from build123d import *

# Parameters (mm, degrees)
F1_DEPTH = 88.9
F2_DEPTH = 6.35
F3_DEPTH = 12.7
F0_W     = 25.2763175084
F0_H     = 38.1


with BuildPart() as f1:
    # F0 (on Front) → F1 (new body, symmetric)
    with BuildSketch(Plane.XZ):
        Polygon((31.75, 22.225), (-50.8, 22.225), (-50.8, -22.225), (50.8, -22.225), (50.8, 22.225), align=None)
    extrude(amount=F1_DEPTH, both=True)

    # F0 (on Front) → F2 (join, symmetric)
    with BuildSketch(Plane.XZ):
        with BuildLine():
            add(Edge.make_bspline(
                [(-50.8, 22.225), (-50.420176295, 53.6387471007), (-0.3042402085, 78.7179242207), (69.217346781, 79.3697470119)],
                knots=[0, 0, 0, 0, 133.0977115432, 133.0977115432, 133.0977115432, 133.0977115432], degree=3))
            Line((-50.8, 22.225), (31.75, 22.225))
            Line((31.75, 22.225), (31.75, 41.275))
            ThreePointArc((31.75, 41.275), (42.6864758578, 67.9911553405), (69.217346781, 79.3697470119))
        make_face()
    extrude(amount=F2_DEPTH, both=True)

    # F0 (on Front) → F3 (join, symmetric)
    with BuildSketch(Plane.XZ):
        with BuildLine():
            Line((31.75, 41.275), (31.75, 22.225))
            Line((31.75, 22.225), (50.8, 22.225))
            Line((50.8, 22.225), (50.8, 41.275))
            ThreePointArc((50.8, 41.275), (56.3796158184, 54.7453841816), (69.85, 60.325))
            Line((69.85, 60.325), (93.4907073213, 60.325))
            Line((93.4907073213, 60.325), (93.4907073213, 79.375))
            Line((93.4907073213, 79.375), (69.85, 79.375))
            add(Edge.make_bspline(
                [(69.217346781, 79.3697470119), (69.4280532127, 79.3717225603), (69.6389379005, 79.3734737242), (69.85, 79.375)],
                knots=[133.0977115432, 133.0977115432, 133.0977115432, 133.0977115432, 133.5011048643, 133.5011048643, 133.5011048643, 133.5011048643], degree=3))
            ThreePointArc((69.217346781, 79.3697470119), (42.6864758578, 67.9911553405), (31.75, 41.275))
        make_face()
        Polygon((118.732270607, 79.375), (93.4907073213, 79.375), (93.4907073213, 60.325), (119.0067035424, 60.325), align=None)
    extrude(amount=F3_DEPTH, both=True)

    # F0 (on Front) → F4 (revolve)
    with BuildSketch(Plane.XZ):
        with Locations((131.6525485671, 70.3345479765)):
            Rectangle(F0_W, F0_H)
    revolve(axis=Axis((119.0143898129, 0, 70.3345479765), (0, 0, 1)))


solid = f1.part
Work out the finished part from the listing and answer in its coordinate system (mm). A direction names the side the tool comes from. Round coordinates to 2 decimals unless told otherwise and drop trailing zeros. Order: outer loops, then holes, each group sorted by start corner. A loop starts at its lowest first (then second) coordinate and runs counter-clockwise, first axis right, second up. Notation, with made-up numbers: M -26.75,3.5 L 4.25,3.5 A33 ccw 4.25,39.5 Z; hole C 51.5,50.5 d10. An arc over 180 degrees is marked long. Put each result on its own line as item: value. Start each with the question number.
Q1. Section A-A, the plane x = 78 is taken. Write down the section's boundary in (y, z) (3 decimals).
Q2. Flat-ended cylindrical pins translate along their axes: pin 1 (8 mm diameter, centred on x = 56.5, y = -37, fed in from +Z); pin 2 (1.9 mm diameter, centred on y = -10.5, z = 33, fed in from -X); pin 3 (25 mm diameter, centred on x = 24, y = 27, fed in from +Z) (3 decimals); pin 4 (7.5 mm diameter, centred on x = 78.5, y = 1.5, fed in from +Z) (3 decimals). Find the tip coordinate at first contact, or state that the pin passes through.
Q3. A tool of negligible diameter and unlimited length cuts with its end or side. For faces 1 (the flat face through (119, 0, 51.285)), 2 (the cylindrical face through (56.232, -0.178, 54.596)), 3 (the flat face through (31.75, 9, 32)), 4 (the flat face through (-1, 88.9, 0)), 5 (the cylindrical face through (42.979, -9.569, 68.285)), from which of +Z, -Z, +X, -X, +Y, -Y can it reach the whole face along a straight path? Write none if from no direction.
Q4. Section B-B, the plane z = 16 is taken. Write down the section's boundary in (x, y).
Q5. Straight lines are drawn through the part: L1, parallel to X at y = -29, z = 4; L2, parallel to Y at x = 71, z = 77; L3, parallel to Z at x = -7, y = 68 (3 decimals). For each, find the intervals that lie inside material, in ascending order. Write a range as [from, to].
Findings below:
1. outline: M -12.7,60.325 L 12.7,60.325 L 12.7,79.375 L -12.7,79.375 Z
2. pin 1: passes through
2. pin 2: stops at x = 31.75
2. pin 3: stops at z = 22.225
2. pin 4: stops at z = 79.375
3. face 1: -Z, +X, +Y, -Y
3. face 2: -Z, +Y, -Y
3. face 3: +Z, -X, +Y
3. face 4: +Z, -Z, +X, -X, +Y
3. face 5: +Z, -X, -Y
4. outline: M -50.8,-88.9 L 50.8,-88.9 L 50.8,88.9 L -50.8,88.9 Z
5. L1: x = [-50.8, 50.8]
5. L2: y = [-12.7, 12.7]
5. L3: z = [-22.225, 22.225]
